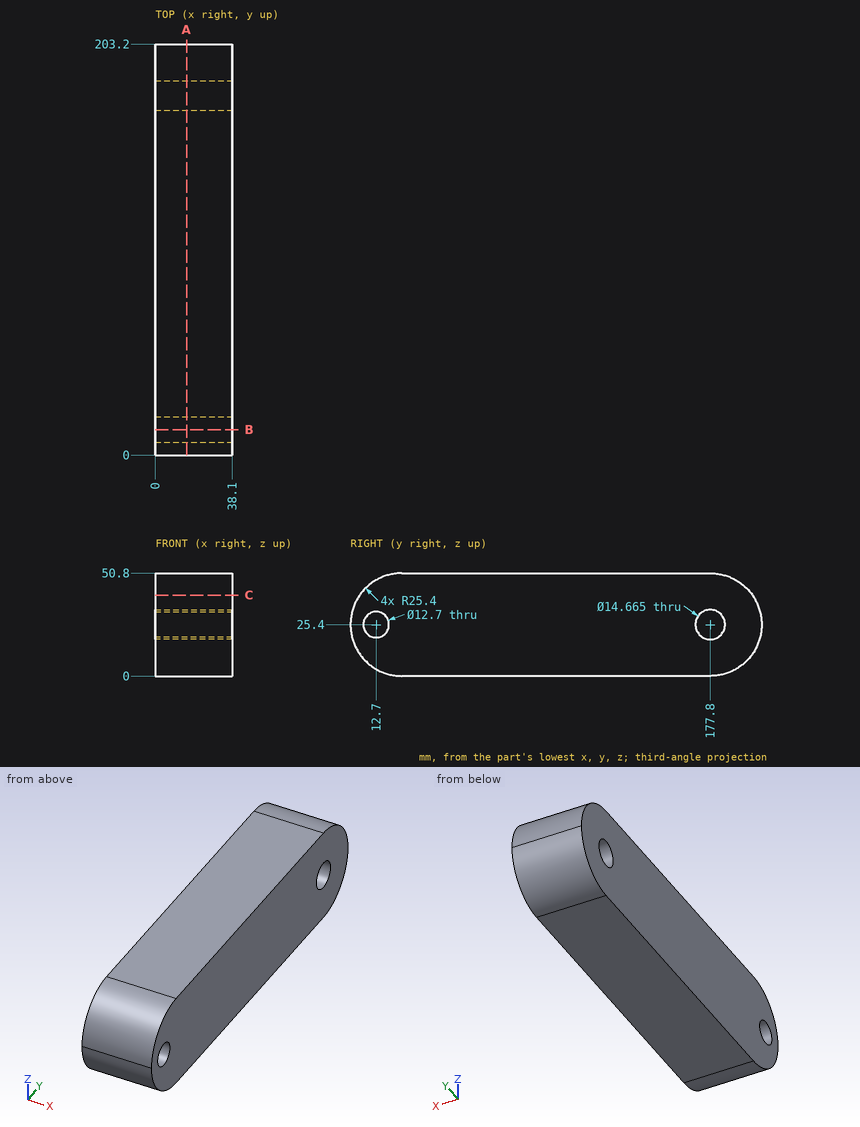
Can you work these out from the drawing? Everything is in mm from the part's minimum corner. Coordinates: 2 decimals unless noted, no trailing zeros. Order: outer loops, then holes, each group sorted by start corner. A loop starts at its lowest first (then second) coordinate and runs counter-clockwise, first axis right, second up. Notation, with made-up numbers: (-30, 29.5) -> (23, 29.5) arc R13 cw to (23, 46.5) -> close; hole circle Ø1 at (46.25, 30.5). An arc over 180 degrees is marked (long way). Return JSON: item names as keys, results as strings.
1) I'm going to push a flat-ended pin straight in: P1, Ø10, axis at x = 25, z = 29, coming from the +Y side. Where does the tip first touch, or does it pass through?
Conclusion:
{"P1": "stops at y = 203.2"}
2) If we section it at B-B on y = 12.7: List the corners of the cut face in (x, z) for me.
Conclusion:
{"outline": "(0, 3.4) -> (38.1, 3.4) -> (38.1, 19.05) -> (0, 19.05) -> close; (0, 31.75) -> (38.1, 31.75) -> (38.1, 47.4) -> (0, 47.4) -> close"}
3) If we section it at A-A on x = 15.5: State how many separate pieces and enclosed holes the cut face has, plus the area to 3 significant figures.
Conclusion:
{"separate pieces": "1", "enclosed holes": "2", "area": "9,470 mm²"}
4) If we section it at C-C on z = 40: List the corners of the cut face in (x, y) for me (1 decimal).
Conclusion:
{"outline": "(0, 4.6) -> (38.1, 4.6) -> (38.1, 198.6) -> (0, 198.6) -> close"}
5) If I drill on probe 1 along Y at (x, z) = (25, 25); probe 2 along Z at (x, y) = (23, 177); probe 3 along Z at (x, y) = (4, 183.5), over which ranges is the centre line in solid material (lowest first)?
Conclusion:
{"probe 1": "y = 0 to 6.36, 19.04 to 170.48, 185.12 to 203.2", "probe 2": "z = 0 to 18.11, 32.69 to 50.8", "probe 3": "z = 0.65 to 20.79, 30.01 to 50.15"}
